Geometry check sheet. Reference: the model listing, model coordinates, mm. Face numbers are marked on the shaded views. A direction names the side the tool comes from. Round coordinates to 2 decimals unless told otherwise and drop trailing zeros. Write each loop counter-clockwise with the first axis right and the second up, starting at its lowest first coordinate (ties: lowest second). Pieces come first, ordered by that corner, then holes. Notation, with made-up numbers: (-22.5, 46.25) - (13.5, 46.25) arc R15 cw to (13.5, 63.25) - close; hole circle Ø4 at (-2.75, -0.75). An arc over 180 degrees is marked (long way). Return JSON: item names as keys, results as strings.
Autodesk Inventor part; units mm, degrees
ref_plane "YZ Plane" through (0, 0, 0) normal (1, 0, 0) x (0, 1, 0)
ref_plane "XZ Plane" through (0, 0, 0) normal (0, 1, 0) x (-1, 0, 0)
ref_plane "XY Plane" through (0, 0, 0) normal (0, 0, 1) x (1, 0, 0)
sketch "Esboço1" plane through (0, 0, 0) normal (0, 1, 0) x (-1, 0, 0)
  line L0 (0, 0) -> (-25.5, 0)
  line L1 (-25.5, 0) -> (-25.5, -25.5)
  line L2 (-25.5, -25.5) -> (0, -25.5)
  line L3 (0, -25.5) -> (0, 0)
  line L4 (-6, -19.5) -> (-19.5, -19.5)
  line L5 (-19.5, -19.5) -> (-19.5, -6)
  line L6 (-19.5, -6) -> (-6, -6)
  line L7 (-6, -6) -> (-6, -19.5)
  point P0 (-25.5, -12.75)
  point P1 (-19.5, -12.75)
  point P2 (-12.75, 0)
  point P3 (-12.75, -6)
  point P4 (-6, -12.75)
  dimension "d0" = 6
  dimension "d1" = 6
  dimension "d2" = 6
  dimension "d3" = 6
  dimension "d4" = 13.5
  dimension "d5" = 13.5
extrude "Extrusão1" add sketch "Esboço1" along normal blind 3 contours L4 L5 L6 L7
extrude "Extrusão2" add sketch "Esboço1" along normal blind 37
properties part number "Tampa_fotometro_3DPrint"
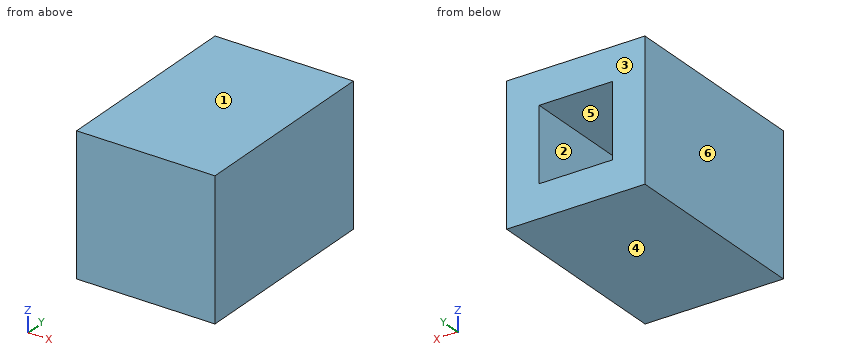
(1) Section check B-B, the plane x = 14. Enter the section's corners in (y, z).
Response values:
{"outline": "(0, -25.5) - (37, -25.5) - (37, -19.5) - (3, -19.5) - (3, -6) - (37, -6) - (37, 0) - (0, 0) - close"}
(2) Section check C-C, the plane z = -10. Enter the section's corners in (x, y).
Response values:
{"outline": "(0, 0) - (25.5, 0) - (25.5, 37) - (19.5, 37) - (19.5, 3) - (6, 3) - (6, 37) - (0, 37) - close"}
(3) Release check for a two-part mould opening along Z. For the marked faces 1, 2, 3 and 4 record: pulls with the +Z half, pulls with the -Z half, needs draft (parallel to the pull), parting line crosses it, or undercut.
Response values:
{"face 1": "pulls with the +Z half", "face 2": "undercut", "face 3": "needs draft", "face 4": "pulls with the -Z half"}
(4) Section check A-A, the plane y = 17.5. Enter the section's corners in (x, z).
Response values:
{"outline": "(0, -25.5) - (25.5, -25.5) - (25.5, 0) - (0, 0) - close; hole (6, -19.5) - (19.5, -19.5) - (19.5, -6) - (6, -6) - close"}
(5) Gauge pin test, flat end, axial feed: pin 1 (1 mm diameter, centred on x = 14, z = -13, fed in from +Y). Record the tip position at first contact, or that the pin passes through.
Response values:
{"pin 1": "stops at y = 3"}
(6) Access from +Z, -Z, +X, -X, +Y, -Y to the whole of each face (thin tool, end or side, straight path). Record for the marked faces 5 and 6.
Response values:
{"face 5": "+Y", "face 6": "+Z, -Z, -X, +Y, -Y"}
(7) Material ranges on line 1 along Z through (x, y) = (17.5, 28); line 2 along X through (y, z) = (25, -12.5); line 3 along Y through (x, z) = (15, -8.5), recorded low to high. Write a range as [from, to].
Response values:
{"line 1": "z = [-25.5, -19.5], [-6, 0]", "line 2": "x = [0, 6], [19.5, 25.5]", "line 3": "y = [0, 3]"}
